Design review of the part shown in the three views and the two pictorial views. Dimensions are in mm from the part's minimum x, y and z. A direction names the side the tool comes from. Give positions to 0.01 mm unless a question says otherwise; leave off trailing zeros. Loops run counter-clockwise (first coordinate to the right, second up) from the corner with the lowest first, then second, coordinate; pieces in that order, holes last.
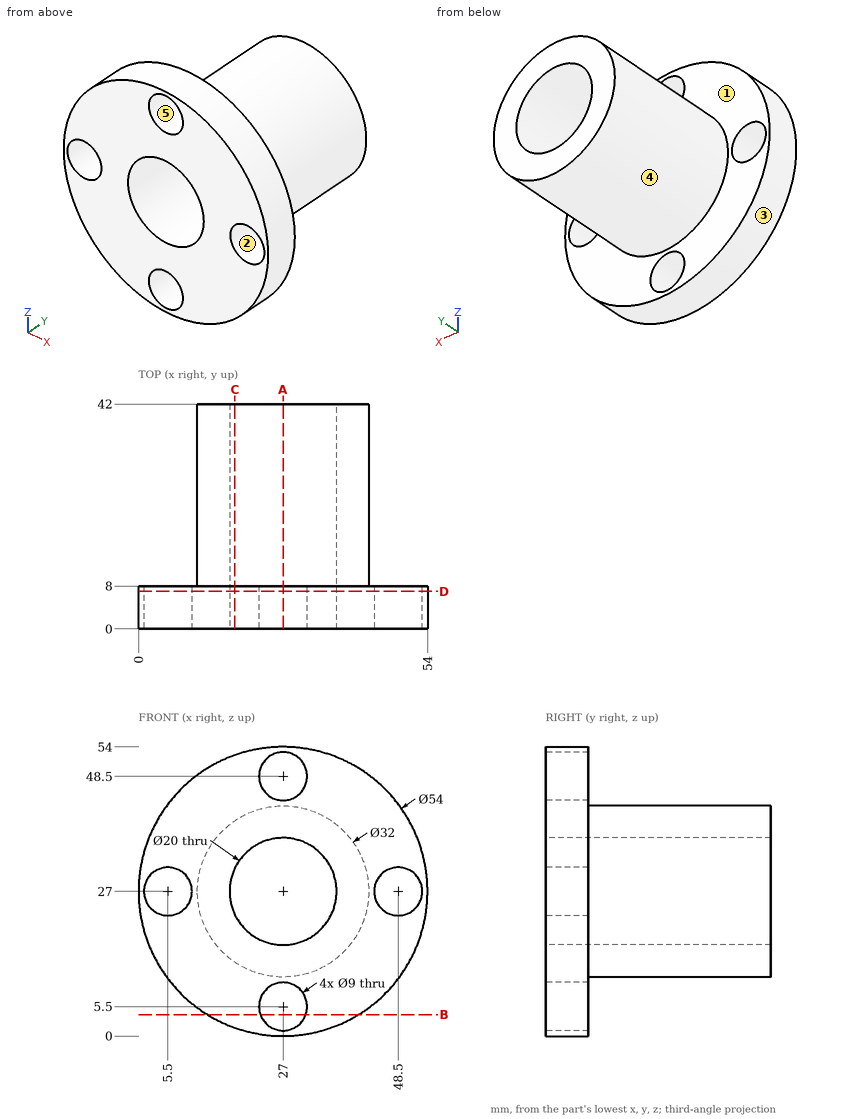
Q1. For pin 1 Ø4 at (y, z) = (19.5, 14.5) entering from -X; pin 2 Ø1.5 at (x, y) = (34.5, 34) entering from -Z; pin 3 Ø5 at (y, z) = (13, 29) entering from +X; pin 4 Ø5 at (x, z) = (15, 44.5) entering from -Y, all flat-tipped, find the tip position at first contact; note any pin that passes through.
Answers:
pin 1: stops at x = 14.93
pin 2: stops at z = 12.49
pin 3: stops at x = 43
pin 4: stops at y = 0
Q2. For probe 1 along X at (y, z) = (2, 31); probe 2 along Z at (x, y) = (27, 28); probe 3 along Y at (x, z) = (10, 13), list the stretches that pass through material, from the lowest coordinate up.
Answers:
probe 1: x = 0.3 to 3.44, 7.56 to 17.83, 36.17 to 46.44, 50.56 to 53.7
probe 2: z = 11 to 17, 37 to 43
probe 3: y = 0 to 8
Q3. Mouldability with a two-part tool opening along X and no side actions: class the marked faces 1, 2 and 3 as +X half, -X half, draft (parallel to the pull), parting line (faces both ways), or undercut.
Answers:
face 1: draft
face 2: undercut
face 3: parting line
Q4. Consider section B-B on z = 4. Give the boundary of the cut face in (x, y), plus the area to 3 significant figures.
Answers:
outline: (12.86, 0) - (22.76, 0) - (22.76, 8) - (12.86, 8) - close; (31.24, 0) - (41.14, 0) - (41.14, 8) - (31.24, 8) - close
area: 158 mm2
Q5. Consider section C-C on x = 18. Give the boundary of the cut face in (y, z).
Answers:
outline: (0, 1.54) - (8, 1.54) - (8, 13.77) - (42, 13.77) - (42, 22.64) - (0, 22.64) - close; (0, 31.36) - (42, 31.36) - (42, 40.23) - (8, 40.23) - (8, 52.46) - (0, 52.46) - close
Q6. Machinability: for the marked faces 4 and 5, which of the approach directions +Z, -Z, +X, -X, +Y, -Y give a long, thin tool a straight path to every point of the face, cutting with its end or side? Answer none if there is none.
Answers:
face 4: +Y
face 5: +Y, -Y
Q7. Consider section D-D on y = 7. Give the boundary of the cut face in (x, z).
Answers:
outline: circle Ø54 at (27, 27); hole circle Ø9 at (5.5, 27); hole circle Ø20 at (27, 27); hole circle Ø9 at (27, 5.5); hole circle Ø9 at (27, 48.5); hole circle Ø9 at (48.5, 27)
Q8. Consider section A-A on x = 27. Give the boundary of the cut face in (y, z), plus the area to 3 significant figures.
Answers:
outline: (0, 0) - (8, 0) - (8, 1) - (0, 1) - close; (0, 10) - (8, 10) - (8, 11) - (42, 11) - (42, 17) - (0, 17) - close; (0, 37) - (42, 37) - (42, 43) - (8, 43) - (8, 44) - (0, 44) - close; (0, 53) - (8, 53) - (8, 54) - (0, 54) - close
area: 536 mm2
